Could you check a few things on this model? Use its own coordinates, in mm. Face numbers are marked on the shaded views. Coordinates: 2 decimals unless noted, no trailing zeros. Order: outer loops, then holes, each group sorted by start corner. A loop starts at its lowest first (then second) coordinate and runs counter-clockwise, first axis right, second up. Notation, with made-up numbers: M -38,-24.75 L -27,-24.75 A17 ccw -27,-15.75 Z; hole C -6,48.25 d4. An arc over 180 degrees is marked long. Put each result on its own line as item: value. Start each with the question number.
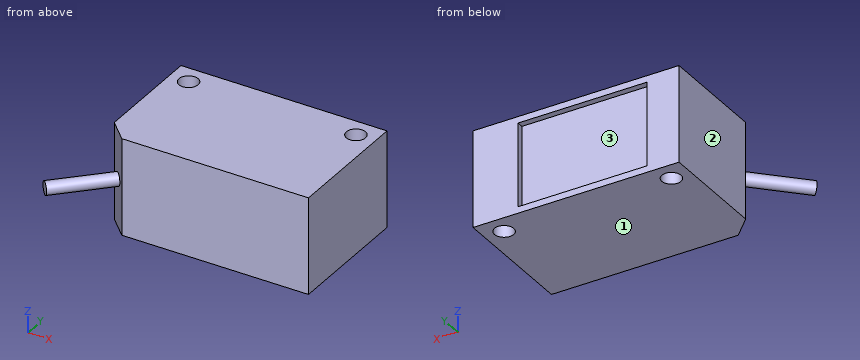
```python
from build123d import *

# Parameters (mm, degrees)
ESQUISSE2_W             = 32
ESQUISSE2_H             = 20
BOSS_EXTRU_1_DEPTH      = 15
ESQUISSE3_R             = 1.5
ENL_V_MAT_EXTRU_1_DEPTH = 15
CHANFREIN1_SIZE         = 3
ESQUISSE5_R             = 1
BOSS_EXTRU_2_DEPTH      = 10
ESQUISSE6_W             = 20
ESQUISSE6_H             = 13
ENL_V_MAT_EXTRU_2_DEPTH = 1


with BuildPart() as part:
    # Esquisse2 → Boss.-Extru.1 (new body)
    with BuildSketch(Plane.XY):
        Rectangle(ESQUISSE2_W, ESQUISSE2_H)
    extrude(amount=BOSS_EXTRU_1_DEPTH)

    # Esquisse3 → Enlèv. mat.-Extru.1 (cut)
    with BuildSketch(Plane.XY.offset(15)):
        with Locations((-13, 7)):
            Circle(ESQUISSE3_R)
    enl_v_mat_extru_1 = extrude(amount=-ENL_V_MAT_EXTRU_1_DEPTH, mode=Mode.SUBTRACT)

    # Symétrie1: Enlèv. mat.-Extru.1 across plane
    add(enl_v_mat_extru_1.mirror(Plane(origin=(0, 0, 0), x_dir=(0, 0, 1), z_dir=(1, 0, 0))), mode=Mode.SUBTRACT)

    # Chanfrein1
    chanfrein1_edges = [part.edges().sort_by_distance(p)[0] for p in [
        (-16, -10, 7.5),
    ]]
    chamfer(chanfrein1_edges, length=CHANFREIN1_SIZE)

    # Esquisse5 → Boss.-Extru.2 (add)
    with BuildSketch(Plane(origin=(-11.5, -11.5, 0), x_dir=(0, 0, 1), z_dir=(-0.707106781, -0.707106781, 0))):
        with Locations((7.5, 4.241320344)):
            Circle(ESQUISSE5_R)
    extrude(amount=BOSS_EXTRU_2_DEPTH)

    # Esquisse6 → Enlèv. mat.-Extru.2 (cut)
    with BuildSketch(Plane(origin=(0, 10, 0), x_dir=(1, 0, 0), z_dir=(0, 1, 0))):
        with Locations((-1, -7.5)):
            Rectangle(ESQUISSE6_W, ESQUISSE6_H)
    extrude(amount=-ENL_V_MAT_EXTRU_2_DEPTH, mode=Mode.SUBTRACT)


solid = part.part
```
Item 1: If we mould it in two halves opening along Z, with no side actions, what happens to the marked faces 1, 2 and 3? For each: released by +Z, released by -Z, zero draft, split by the parting line, or undercut.
Item 2: I need wall thicknesses on probe 1 along Y at (x, z) = (-13, 4.5); probe 2 along Y at (x, z) = (-9, 4); probe 3 along Y at (x, z) = (10, 1.75). Which ranges of each line are inside material? Lowest first, please.
Item 3: For pin 1 Ø4 at (y, z) = (3.5, 12) entering from -X; pin 2 Ø3 at (x, z) = (11, 10.5) entering from -Y, each with a flat end and sliding along its axis, tell me the tip position at first contact or that it passes through.
Item 4: If we section it at B-B on x = 13: Write out the boundary of the cut face in (y, z).
Item 5: If we section it at D-D on x = -6: Write out the boundary of the cut face in (y, z), then the cut area to 3 significant figures.
Item 6: If we section it at A-A on y = 7: Write out the boundary of the cut face in (x, z), then the cut area to 3 significant figures.
Item 7: If we section it at C-C on z = 9.5: Write out the boundary of the cut face in (x, y), then the cut area to 3 significant figures.
Geometry check:
1. face 1: released by -Z
1. face 2: zero draft
1. face 3: undercut
2. probe 1: y = -10 to 5.5, 8.5 to 10
2. probe 2: y = -10 to 9
2. probe 3: y = -10 to 10
3. pin 1: stops at x = -16
3. pin 2: stops at y = -10
4. outline: M -10,0 L 5.5,0 L 5.5,15 L -10,15 Z; M 8.5,0 L 10,0 L 10,15 L 8.5,15 Z
5. outline: M -10,0 L 10,0 L 10,1 L 9,1 L 9,14 L 10,14 L 10,15 L -10,15 Z
5. area: 287 mm²
6. outline: M -16,0 L -14.5,0 L -14.5,15 L -16,15 Z; M -11.5,0 L 11.5,0 L 11.5,15 L -11.5,15 Z; M 14.5,0 L 16,0 L 16,15 L 14.5,15 Z
6. area: 390 mm²
7. outline: M -16,-7 L -13,-10 L 16,-10 L 16,10 L 9,10 L 9,9 L -11,9 L -11,10 L -16,10 Z; hole C -13,7 d3; hole C 13,7 d3
7. area: 601 mm²
